Read the model definition and answer for the solid it produces. Units are mm, in the model's axes. A direction names the side the tool comes from. Coordinates: 2 decimals unless noted, no trailing zeros. Write each loop counter-clockwise with the first axis right and the second up, starting at its lowest first coordinate (ties: lowest second). Pieces come first, ordered by that corner, then holes. Notation, with made-up numbers: (-25, 74) - (-4, 74) arc R20 ccw to (-4, 104) - close; hole circle Ø9 at (68.5, -24.75). An arc over 180 degrees is marked (long way). Return JSON: item names as keys, results as strings.
```python
from build123d import *

# Parameters (mm, degrees)
SKETCH1_W                 = 17.78
SKETCH1_H                 = 40.64
PCB_DEPTH                 = 1.5748
SKETCH2_R                 = 0.381
HOLE_PATTERN_SEED_1_DEPTH = 1.5748
HP_1X16_COUNT             = 16
HP_1X16_PITCH             = 2.54
SKETCH3_R                 = 0.381
HOLE_PATTERN_SEED_2_DEPTH = 1.5748
HP_1X08_COUNT             = 8
HP_1X08_PITCH             = 2.54
SKETCH4_W                 = 8.5598
SKETCH4_H                 = 3.81
SSOP_24_DEPTH             = 1.35128


with BuildPart() as part:
    # Sketch1 → PCB (new body)
    with BuildSketch(Plane(origin=(0, 0, 0), x_dir=(1, 0, 0), z_dir=(0, 1, 0))):
        with Locations((8.89, 20.32)):
            Rectangle(SKETCH1_W, SKETCH1_H)
    extrude(amount=PCB_DEPTH)

    # Sketch2 → Hole Pattern seed 1 (cut)
    with BuildSketch(Plane(origin=(0, 1.5748, 0), x_dir=(1, 0, 0), z_dir=(0, 1, 0))):
        with Locations((1.27, 1.27)):
            Circle(SKETCH2_R)
    hole_pattern_seed_1 = extrude(amount=-HOLE_PATTERN_SEED_1_DEPTH, mode=Mode.SUBTRACT)

    # HP 1x16: Hole Pattern seed 1 ×16
    with Locations(*[(0, 0, -i * HP_1X16_PITCH) for i in range(1, HP_1X16_COUNT)]):
        add(hole_pattern_seed_1, mode=Mode.SUBTRACT)

    # Sketch3 → Hole Pattern seed 2 (cut)
    with BuildSketch(Plane(origin=(0, 1.5748, 0), x_dir=(1, 0, 0), z_dir=(0, 1, 0))):
        with Locations((16.51, 11.43)):
            Circle(SKETCH3_R)
    hole_pattern_seed_2 = extrude(amount=-HOLE_PATTERN_SEED_2_DEPTH, mode=Mode.SUBTRACT)

    # HP 1x08: Hole Pattern seed 2 ×8
    with Locations(*[(0, 0, -i * HP_1X08_PITCH) for i in range(1, HP_1X08_COUNT)]):
        add(hole_pattern_seed_2, mode=Mode.SUBTRACT)

    # Sketch4 → SSOP-24 (add)
    with BuildSketch(Plane(origin=(0, 1.5748, 0), x_dir=(1, 0, 0), z_dir=(0, 1, 0))):
        with Locations((8.89, 20.32)):
            Rectangle(SKETCH4_W, SKETCH4_H)
    extrude(amount=SSOP_24_DEPTH)


solid = part.part
```
(1) Straight lines are drawn through the part: line 1 (X direction, y = 0.4, z = -11.43); line 2 (X direction, y = 1, z = -6.35); line 3 (Y direction, x = 10, z = -31.5). For each, find the intervals that lie inside material, in ascending order. Write a range as from..to.
Answer:
{"line 1": "0..0.89, 1.65..16.13, 16.89..17.78", "line 2": "0..0.89, 1.65..17.78", "line 3": "0..1.57"}
(2) A cutting plane is placed at A-A (z = -1.27). Determine the outline of the cut face in (x, y), and give its area (3 significant figures).
Answer:
{"outline": "(0, 0) - (0.89, 0) - (0.89, 1.57) - (0, 1.57) - close; (1.65, 0) - (17.78, 0) - (17.78, 1.57) - (1.65, 1.57) - close", "area": "26.8 mm²"}
(3) A cutting plane is placed at C-C (y = 0.7). State how many separate pieces and enclosed holes the cut face has, and give its area (3 significant figures).
Answer:
{"separate pieces": "1", "enclosed holes": "24", "area": "712 mm²"}
(4) Flat-ended cylindrical pins translate along their axes: P1, Ø1.1, axis at x = 8, y = 2.5, coming from the -Z side (3 decimals); P2, Ø1, axis at x = 13, z = -7.5, coming from the +Y side; P3, Ø1.1, axis at x = 9, y = 2.5, coming from the +Z side (3 decimals). Find the tip coordinate at first contact, or state that the pin passes through.
Answer:
{"P1": "z = -22.225", "P2": "y = 1.57", "P3": "z = -18.415"}
(5) A cutting plane is placed at D-D (x = 7.25). Determine the outline of the cut face in (y, z) (3 decimals), and give its area (3 significant figures).
Answer:
{"outline": "(0, -40.64) - (1.575, -40.64) - (1.575, -22.225) - (2.926, -22.225) - (2.926, -18.415) - (1.575, -18.415) - (1.575, 0) - (0, 0) - close", "area": "69.1 mm²"}
(6) A cutting plane is placed at B-B (z = -21.59). Determine the outline of the cut face in (x, y).
Answer:
{"outline": "(0, 0) - (0.89, 0) - (0.89, 1.57) - (0, 1.57) - close; (1.65, 0) - (16.13, 0) - (16.13, 1.57) - (13.17, 1.57) - (13.17, 2.93) - (4.61, 2.93) - (4.61, 1.57) - (1.65, 1.57) - close; (16.89, 0) - (17.78, 0) - (17.78, 1.57) - (16.89, 1.57) - close"}
(7) Which of the six approach directions +Z, -Z, +X, -X, +Y, -Y give full straight-line access (tool end or side, diameter ignored) to faces 1 (the face through (9, 2, -22.225)), 2 (the face through (9, 1, -40.64)), 3 (the face through (13.17, 2, -20)), 4 (the face through (4.61, 2, -20)), 5 (the face through (9, 2, -18.415))?
Answer:
{"face 1": "-Z, +X, -X, +Y", "face 2": "-Z, +X, -X, +Y, -Y", "face 3": "+Z, -Z, +X, +Y", "face 4": "+Z, -Z, -X, +Y", "face 5": "+Z, +X, -X, +Y"}
